Design review of the part built by this model. Coordinates are the model's own, in mm. A direction names the side the tool comes from. Give positions to 0.01 mm unless a question says otherwise; leave off trailing zeros. Order: outer loops, then holes, each group sorted by start corner. A loop starts at its lowest first (then second) coordinate and runs counter-clockwise, first axis right, second up. Notation, with made-up numbers: (-24.5, 71) -> (33.5, 71) arc R9 ccw to (33.5, 76) -> close; hole circle Ø10 at (-1.5, 37). An arc over 180 degrees is marked (long way). One line per item, written item: value. Start each with the question number.
1) Consider section A-A (x = -2.5). State the section outline as (y, z) points, plus the area to 3 significant figures.
2) The part is to be moulded in two halves that separate along X. For faces 1 (the face through (0.104, 8.965, 3.699)), 2 (the face through (-8.737, 8.709, 1.521)), 3 (the face through (0.12, -7.94, 0.71)), 4 (the face through (8.709, -8.737, 1.521)), say which applies: released by +X, released by -X, zero draft, split by the parting line, or undercut.
3) Tool access review of faces 5 (the face through (0, -9.25, 1)), 6 (the face through (-7.94, 0.12, 0.71)): name each direction out of +Z, -Z, +X, -X, +Y, -Y from which nothing blocks a thin tool from reaching the whole face with its end or side.
4) Wall thickness on line 1 along Y through (x, z) = (5.5, 1.5); line 2 along Y through (x, z) = (-6, 3.05): over which ranges is each line inside the solid? List them lowest first. Write a range as from..to.
5) For pin 1 (4.5 mm diameter, centred on x = 1.5, y = 3.5, fed in from -Z); pin 2 (2 mm diameter, centred on x = 4.5, y = 7, fed in from -Z), all flat-tipped, find the tip position at first contact; note any pin that passes through.
from build123d import *

# Parameters (mm, degrees)
SCHIZZO1_W                   = 18.5
SCHIZZO1_H                   = 18.5
ESTRUSIONE_ESTRUSIONE1_DEPTH = 4
RACCORDO1_R                  = 1.8
RACCORDO2_R                  = 1
SVUOTA1_T                    = -2
SMUSSO1_SIZE                 = 1.4


with BuildPart() as part:
    # Schizzo1 → Estrusione-Estrusione1 (new body)
    with BuildSketch(Plane.XY):
        Rectangle(SCHIZZO1_W, SCHIZZO1_H)
    extrude(amount=ESTRUSIONE_ESTRUSIONE1_DEPTH)

    # Raccordo1
    raccordo1_edges = [part.edges().sort_by_distance(p)[0] for p in [
        (9.25, -9.25, 2),
        (-9.25, -9.25, 2),
        (-9.25, 9.25, 2),
        (9.25, 9.25, 2),
    ]]
    fillet(raccordo1_edges, radius=RACCORDO1_R)

    # Raccordo2
    raccordo2_edges = [part.edges().sort_by_distance(p)[0] for p in [
        (-9.25, 0, 4),
        (0, 9.25, 4),
        (9.25, 0, 4),
        (0, -9.25, 4),
        (8.722792206, 8.722792206, 4),
        (8.722792206, -8.722792206, 4),
        (-8.722792206, -8.722792206, 4),
        (-8.722792206, 8.722792206, 4),
    ]]
    fillet(raccordo2_edges, radius=RACCORDO2_R)

    # Svuota1
    svuota1_openings = [part.faces().sort_by_distance(p)[0] for p in [
        (0, 0, 0),
    ]]
    offset(amount=SVUOTA1_T, openings=svuota1_openings, kind=Kind.INTERSECTION)

    # Smusso1
    smusso1_edges = [part.edges().sort_by_distance(p)[0] for p in [
        (7.25, 0, 0),
        (0, 7.25, 0),
        (-7.25, 0, 0),
        (0, -7.25, 0),
    ]]
    chamfer(smusso1_edges, length=SMUSSO1_SIZE)


solid = part.part
Checked values:
1. outline: (-9.25, 0) -> (-8.65, 0) -> (-7.25, 1.4) -> (-7.25, 2) -> (7.25, 2) -> (7.25, 1.4) -> (8.65, 0) -> (9.25, 0) -> (9.25, 3) arc R1 ccw to (8.25, 4) -> (-8.25, 4) arc R1 ccw to (-9.25, 3) -> close
1. area: 42.6 mm^2
2. face 1: zero draft
2. face 2: released by -X
2. face 3: undercut
2. face 4: released by +X
3. face 5: +Z, -Z, +X, -X, -Y
3. face 6: -Z
4. line 1: y = -9.25..-7.25, 7.25..9.25
4. line 2: y = -9.25..9.25
5. pin 1: stops at z = 2
5. pin 2: stops at z = 0.65
